Study the drawing (mm; zero at the part's minimum x, y, z) and answer. A direction names the side the tool comes from. Round coordinates to 2 decimals unless told otherwise and drop trailing zeros. Loops run counter-clockwise (first coordinate to the right, second up) from the corner with the lowest first, then second, coordinate; pieces in that order, holes last. Notation, with made-up numbers: (22.25, 75.5) - (29.25, 75.5) arc R16 cw to (29.25, 79.5) - close; hole circle Ø4 at (1, -10.75). An arc over 180 degrees is marked (long way). One line per item, written item: value.
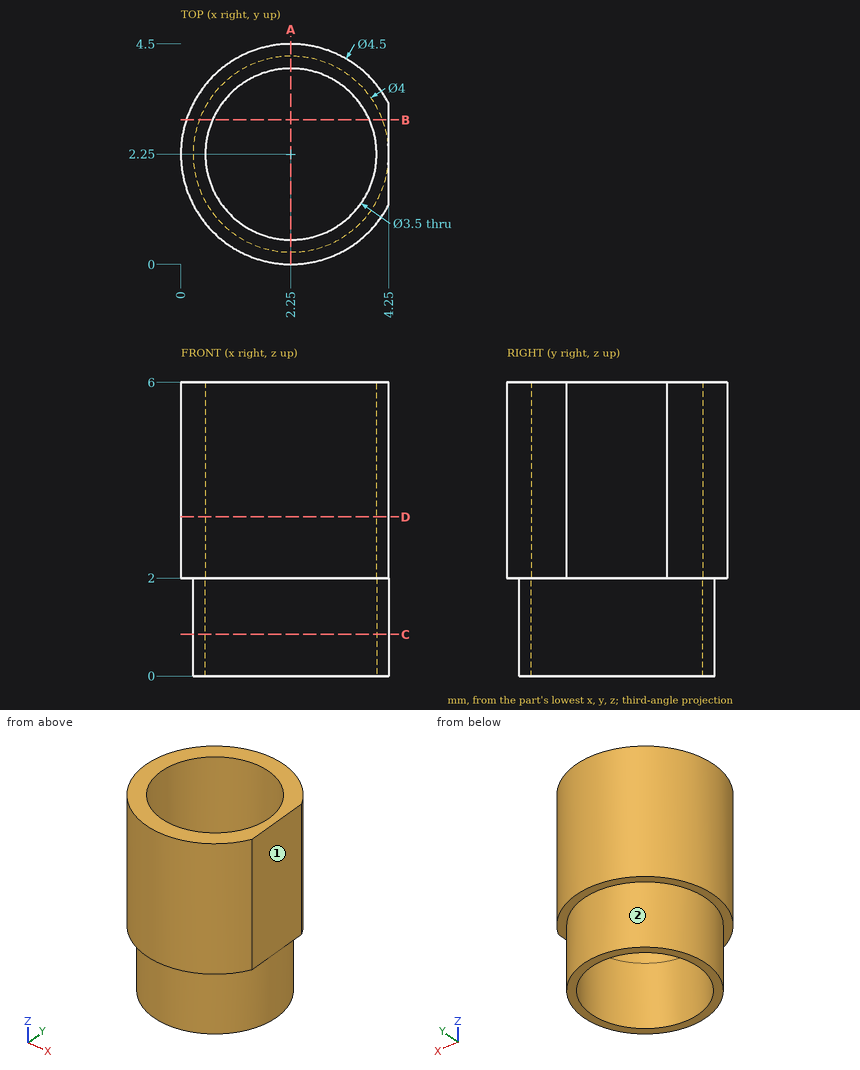
1) A cutting plane is placed at B-B on y = 2.95. Give the vertices of the cut face in (x, z).
Final values:
outline: (0.11, 2) - (0.38, 2) - (0.38, 0) - (0.65, 0) - (0.65, 6) - (0.11, 6) - close; (3.85, 0) - (4.12, 0) - (4.12, 2) - (4.25, 2) - (4.25, 6) - (3.85, 6) - close
2) Consider L1, parallel to Y at x = 2.25, z = 4.95; L2, parallel to Y at x = 2.25, z = 1.65; L3, parallel to X at y = 2.25, z = 3.35. Determine where each line is inside the solid, lowest interval first.
Final values:
L1: 0 to 0.5, 4 to 4.5
L2: 0.25 to 0.5, 4 to 4.25
L3: 0 to 0.5, 4 to 4.25
3) A cutting plane is placed at D-D on z = 3.25. Give the vertices of the cut face in (x, y), and give its area (3 significant figures).
Final values:
outline: (4.25, 1.22) - (4.25, 3.28) arc R2.25 ccw (long way) to start; hole circle Ø3.5 at (2.25, 2.25)
area: 5.94 mm2
4) A cutting plane is placed at C-C on z = 0.85. Give the vertices of the cut face in (x, y), and give its area (3 significant figures).
Final values:
outline: circle Ø4 at (2.25, 2.25); hole circle Ø3.5 at (2.25, 2.25)
area: 2.95 mm2
5) A cutting plane is placed at A-A on x = 2.25. Give the vertices of the cut face in (y, z).
Final values:
outline: (0, 2) - (0.25, 2) - (0.25, 0) - (0.5, 0) - (0.5, 6) - (0, 6) - close; (4, 0) - (4.25, 0) - (4.25, 2) - (4.5, 2) - (4.5, 6) - (4, 6) - close
6) For the marked faces 1 and 2, determine the directions among +Z, -Z, +X, -X, +Y, -Y from which every point of the face is accessible in a straight line to the end or side of a thin tool.
Final values:
face 1: +Z, -Z, +X, +Y, -Y
face 2: -Z
7) This flat-tipped pin is pushed along its axis until it touches: pin 1 Ø2 at (x, y) = (2.25, 2.25) entering from -Z. Where does it stop, or does it pass through?
Final values:
pin 1: through
